Input: part model. Units: mm. Frame: model coordinates. Face numbers are marked on the shaded views. A direction names the side the tool comes from. Round coordinates to 2 decimals unless told otherwise and drop trailing zeros. Loops run counter-clockwise (first coordinate to the right, second up) from the corner with the lowest first, then second, coordinate; pieces in that order, holes last. Notation, with made-up numbers: (72, -25) -> (102, -25) arc R20 cw to (102, 13) -> close; hole circle Ø6 at (-12, 24.25). An arc over 180 degrees is marked (long way). One line per question, with ' | ' between items. Start each with the question number.
Q1. Access query for the marked faces 4 and 5. Directions: +Z, -Z, +X, -X, +Y, -Y. A direction counts if a zero-diameter tool reaches every point of the face in a straight line with its end or side. Return the directions, or none.
Q2. Mould query, pull axis X, two halves, no side actions, for the marked faces 1, 2 and 3. Classes: pulls with the +X half, pulls with the -X half, needs draft (parallel to the pull), parting line crosses it, or undercut.
Q3. Material intervals for L1, parallel to Y at x = 0, z = -0.25; L2, parallel to Y at x = 0, z = -4.5; L3, parallel to X at y = -1.25, z = -4.75, sorted ascending.
Q4. Cut plane C-C on z = 0.5. Return loops of the section in (x, y).
Q5. Cut plane D-D on y = -7.25. Return loops of the section in (x, z), and give its area (3 significant figures).
Q6. Contact query for flat-ended pins moving along their axis: P1, Ø5, axis at y = 3.5, z = -0.5, coming from the -X side; P2, Ø9, axis at x = 1, y = -3, coming from the +Z side; P3, Ø2, axis at x = 5, z = -5, coming from the -Y side; P4, Ø5, axis at x = 6, z = -2.5, coming from the -Y side. Output: stop coordinate, or through.
Q7. Cut plane A-A on x = 0. Return loops of the section in (y, z).
from build123d import *

# Parameters (mm, degrees)
F0_R     = 7.95
F1_DEPTH = 3
F2_R     = 8.75
F3_DEPTH = 3.5
F4_R     = 7.95
F5_DEPTH = 3
F7_D     = 6.6


with BuildPart() as f1:
    # F0 (on Top) → F1 (new body)
    with BuildSketch(Plane.XY):
        Circle(F0_R)
    extrude(amount=F1_DEPTH)

    # F2 (on face) → F3 (join)
    with BuildSketch(Plane(origin=(0, 0, 0), x_dir=(1, 0, 0), z_dir=(0, 0, -1))):
        Circle(F2_R)
    extrude(amount=F3_DEPTH)

    # F4 (on face) → F5 (join)
    with BuildSketch(Plane(origin=(0, 0, -3.5), x_dir=(1, 0, 0), z_dir=(0, 0, -1))):
        Circle(F4_R)
    extrude(amount=F5_DEPTH)

    # F7 (through all)
    with Locations(Plane.XY.offset(3)):
        with Locations((0, 0)):
            Hole(F7_D / 2)


solid = f1.part
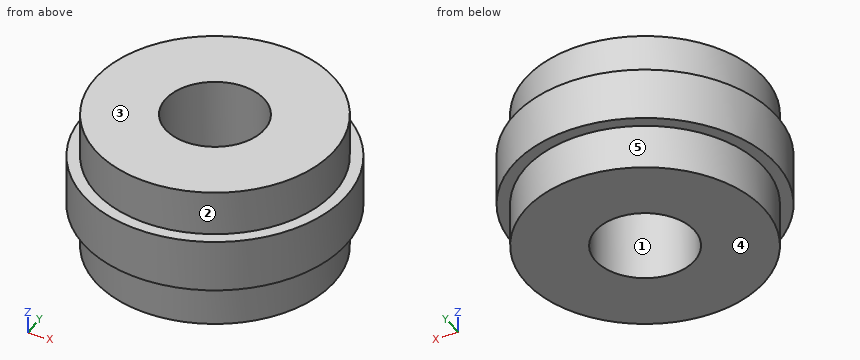
Results:
1) face 4: -Z, +X, -X, +Y, -Y | face 5: -Z
2) face 1: undercut | face 2: parting line crosses it | face 3: needs draft
3) L1: -8.75 to -3.3, 3.3 to 8.75 | L2: -7.95 to -3.3, 3.3 to 7.95 | L3: -7.85 to -3.05, 3.05 to 7.85
4) outline: circle Ø15.9 at (0, 0); hole circle Ø6.6 at (0, 0)
5) outline: (-4.9, -3.5) -> (-3.26, -3.5) -> (-3.26, -6.5) -> (3.26, -6.5) -> (3.26, -3.5) -> (4.9, -3.5) -> (4.9, 0) -> (3.26, 0) -> (3.26, 3) -> (-3.26, 3) -> (-3.26, 0) -> (-4.9, 0) -> close | area: 73.4 mm^2
6) P1: x = -8.69 | P2: z = 3 | P3: y = -6.87 | P4: y = -8.02
7) outline: (-8.75, -3.5) -> (-7.95, -3.5) -> (-7.95, -6.5) -> (-3.3, -6.5) -> (-3.3, 3) -> (-7.95, 3) -> (-7.95, 0) -> (-8.75, 0) -> close; (3.3, -6.5) -> (7.95, -6.5) -> (7.95, -3.5) -> (8.75, -3.5) -> (8.75, 0) -> (7.95, 0) -> (7.95, 3) -> (3.3, 3) -> close
